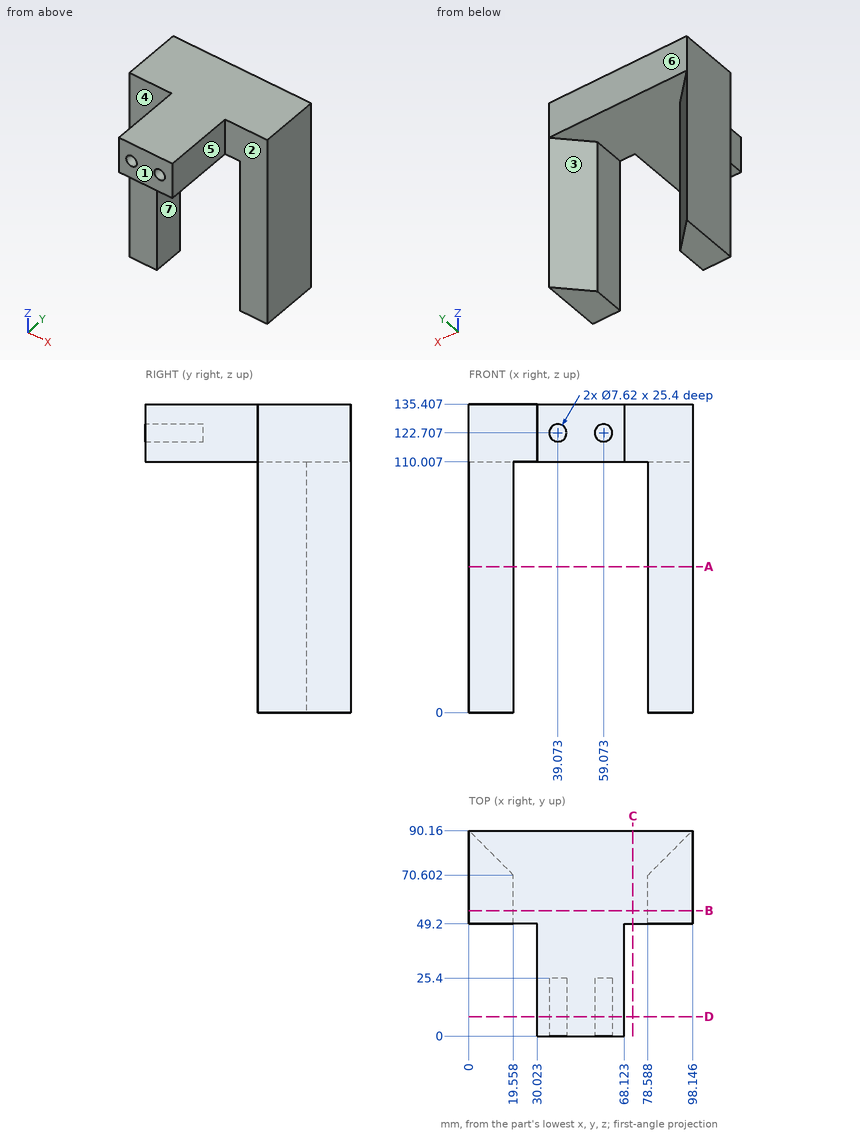
Answer from the drawing. Dimensions are ordinates in mm from the lowest x, y and z of the part. A direction names the side the tool comes from. Give positions to 0.01 mm unless a question says otherwise; leave off trailing zeros. Loops run counter-clockwise (first coordinate to the right, second up) from the corner with the lowest first, then second, coordinate; pieces in that order, holes last. Notation, with made-up numbers: (83.5, 60) - (98.5, 60) arc R22 cw to (98.5, 99) - close; hole circle Ø3 at (86, 32). An arc over 180 degrees is marked (long way). Answer as a JSON object with one key per item and string values.
1. Find the intervals of material crossed by L1, parallel to X at y = 60.5, z = 102.5 (1 decimal); L2, parallel to X at y = 45, z = 129; L3, parallel to Y at x = 88.5, z = 120.5, in increasing order. Write a range as [from, to].
Determined:
{"L1": "[0, 19.6], [78.6, 98.1]", "L2": "[30.02, 68.12]", "L3": "[49.2, 90.16]"}
2. A cutting plane is placed at D-D (y = 8.5). Write down the section's boundary in (x, z).
Determined:
{"outline": "(30.02, 110.01) - (68.12, 110.01) - (68.12, 135.41) - (30.02, 135.41) - close; hole circle Ø7.62 at (39.07, 122.71); hole circle Ø7.62 at (59.07, 122.71)"}
3. For the marked faces 1, 2, 3 and 4, determine the directions among +Z, -Z, +X, -X, +Y, -Y from which every point of the face is accessible in a straight line to the end or side of a thin tool.
Determined:
{"face 1": "+Z, -Z, +X, -X, -Y", "face 2": "+Z, -Z, +X, -Y", "face 3": "-Z, +Y", "face 4": "+Z, -Z, -X, -Y"}
4. A cutting plane is placed at C-C (x = 72). Write down the section's boundary in (y, z).
Determined:
{"outline": "(49.2, 110.01) - (90.16, 110.01) - (90.16, 135.41) - (49.2, 135.41) - close"}
5. For a pull along X with two mould halves and no side action, classify the marked faces 5, 6 and 7 as pulls with the +X half, pulls with the -X half, needs draft (parallel to the pull), parting line crosses it, or undercut.
Determined:
{"face 5": "pulls with the +X half", "face 6": "needs draft", "face 7": "undercut"}
6. A cutting plane is placed at B-B (y = 55). Write down the section's boundary in (x, z) (1 decimal), then the cut area to 3 significant figures.
Determined:
{"outline": "(0, 0) - (19.6, 0) - (19.6, 110) - (78.6, 110) - (78.6, 0) - (98.1, 0) - (98.1, 135.4) - (0, 135.4) - close", "area": "6,800 mm²"}
7. A cutting plane is placed at A-A (z = 64). Write down the section's boundary in (x, y) (1 decimal), then the cut area to 3 significant figures.
Determined:
{"outline": "(0, 49.2) - (19.6, 49.2) - (19.6, 70.6) - (0, 90.2) - close; (78.6, 49.2) - (98.1, 49.2) - (98.1, 90.2) - (78.6, 70.6) - close", "area": "1,220 mm²"}
8. Flat-ended cylindrical pins translate along their axes: pin 1 Ø2.5 at (x, z) = (57.5, 121.5) entering from -Y; pin 2 Ø12.5 at (y, z) = (15, 118) entering from -X; pin 3 Ø2 at (x, z) = (78.5, 73) entering from -Y. Find the tip coordinate at first contact, or state that the pin passes through.
Determined:
{"pin 1": "y = 25.4", "pin 2": "x = 30.02", "pin 3": "y = 49.2"}
